Geometry check sheet. Reference: the model listing, model coordinates, mm. A direction names the side the tool comes from. Give positions to 0.01 mm unless a question says otherwise; leave off trailing zeros. Loops run counter-clockwise (first coordinate to the right, second up) from the corner with the lowest first, then second, coordinate; pieces in that order, holes last. Notation, with made-up numbers: (-23, -9.75) -> (25, -9.75) arc R16 cw to (25, 14.25) -> close; hole circle Ø9 at (67, -37.75). An arc over 180 degrees is marked (long way). Write item = value, one per line.
```python
from build123d import *

# Parameters (mm, degrees)
CUT_EXTRUDE1_DEPTH = 0.635
SKETCH4_R          = 4.7625
CUT_EXTRUDE2_DEPTH = 0.635


with BuildPart() as part:
    # Sketch1 → Revolve1 (revolve)
    with BuildSketch(Plane.XY, mode=Mode.PRIVATE) as revolve1_sk:
        Polygon((-38.1, -2.54), (0, -2.54), (0, 0), (-50.8, 0), (-50.8, -5.08), (-38.1, -5.08), align=None)
    revolve(revolve1_sk.sketch.rotate(Axis((0, 4.567685351, 0), (0, -1, 0)), 270), axis=Axis((0, 4.567685351, 0), (0, -1, 0)))

    # Sketch3 → Cut-Extrude1 (cut)
    with BuildSketch(Plane(origin=(0, 0, 0), x_dir=(1, 0, 0), z_dir=(0, 1, 0))):
        Polygon((-1.833087105, 41.275), (-3.666174209, 38.1), (-1.833087105, 34.925), (1.833087105, 34.925), (3.666174209, 38.1), (1.833087105, 41.275), align=None)
        Polygon((-34.828654989, -15.875), (-36.661742094, -19.05), (-34.828654989, -22.225), (-31.16248078, -22.225), (-29.329393675, -19.05), (-31.16248078, -15.875), align=None)
        Polygon((34.828654989, -15.875), (31.16248078, -15.875), (29.329393675, -19.05), (31.16248078, -22.225), (34.828654989, -22.225), (36.661742094, -19.05), align=None)
    extrude(amount=-CUT_EXTRUDE1_DEPTH, mode=Mode.SUBTRACT)

    # Sketch4 → Cut-Extrude2 (cut)
    with BuildSketch(Plane(origin=(0, 0, 0), x_dir=(1, 0, 0), z_dir=(0, 1, 0))):
        with Locations(Location((32.995567884, -19.05, 0), (0, 0, 270))):
            Circle(SKETCH4_R)
        with Locations(Location((-32.995567884, -19.05, 0), (0, 0, 270))):
            Circle(SKETCH4_R)
        with Locations(Location((0, 38.1, 0), (0, 0, 270))):
            Circle(SKETCH4_R)
    extrude(amount=-CUT_EXTRUDE2_DEPTH, mode=Mode.SUBTRACT)


solid = part.part
```
Item 1: Section check B-B, the plane x = 0. Record the cut outline in (y, z) (1 decimal).
Answer:
outline = (-5.1, -50.8) -> (0, -50.8) -> (0, -42.9) -> (-0.6, -42.9) -> (-0.6, -33.3) -> (0, -33.3) -> (0, 50.8) -> (-5.1, 50.8) -> (-5.1, 38.1) -> (-2.5, 38.1) -> (-2.5, -38.1) -> (-5.1, -38.1) -> close
Item 2: Tool access check on faces 4 (the flat face through (-1, -2.54, -1)), 5 (the cylindrical face through (-35.89, -0.31, 15.27)), 6 (the flat face through (-1, 0, 1)). Record the directions out of +Z, -Z, +X, -X, +Y, -Y that give a thin tool (end or side, any length) a straight path to the whole face; none if there is none.
Answer:
face_4 = -Y
face_5 = +Y
face_6 = +Z, -Z, +X, -X, +Y
Item 3: Draft check along X on faces 1 (the cylindrical face through (36.214, -0.313, 15.54)), 2 (the flat face through (-38, -5.08, 7)), 3 (the cylindrical face through (30.911, -2.576, -40.313)). Enter one of: +X half, -X half, draft (parallel to the pull), parting line (faces both ways), or undercut.
Answer:
face_1 = undercut
face_2 = draft
face_3 = parting line
Item 4: Section check C-C, the plane y = -1.55. Record the cut outline in (x, z).
Answer:
outline = circle Ø101.6 at (0, 0)
Item 5: Section check A-A, the plane z = 0. Record the cut outline in (x, y).
Answer:
outline = (-50.8, -5.08) -> (-38.1, -5.08) -> (-38.1, -2.54) -> (38.1, -2.54) -> (38.1, -5.08) -> (50.8, -5.08) -> (50.8, 0) -> (-50.8, 0) -> close
Item 6: Gauge pin test, flat ends, axial feed: pin 1 (3 mm diameter, centred on x = -31.5, z = 17, fed in from +Y) (3 decimals); pin 2 (1.5 mm diameter, centred on y = -0.5, z = -26, fed in from -X); pin 3 (2 mm diameter, centred on y = -4, z = 29, fed in from +X). Record the tip position at first contact, or that the pin passes through.
Answer:
pin_1 = -0.635
pin_2 = -44.08
pin_3 = 42.39
Item 7: Thickness scan on L1, parallel to X at y = -4.6, z = 0; L2, parallel to X at y = -0.2, z = 19.05; L3, parallel to Y at x = 10.5, z = 13.5. Record the ranges inside material, lowest first. Write a range as [from, to].
Answer:
L1 = [-50.8, -38.1], [38.1, 50.8]
L2 = [-47.09, -37.76], [-28.23, 28.23], [37.76, 47.09]
L3 = [-2.54, 0]
Item 8: Section check D-D, the plane x = 18. Record the cut outline in (y, z).
Answer:
outline = (-5.08, -47.5) -> (0, -47.5) -> (0, 47.5) -> (-5.08, 47.5) -> (-5.08, 33.58) -> (-2.54, 33.58) -> (-2.54, -33.58) -> (-5.08, -33.58) -> close
